For this review, take the finished solid that the model builds, in its own axes (mm). Round coordinates to 2 decimals unless told otherwise and drop trailing zeros. Loops run counter-clockwise (first coordinate to the right, second up) from the corner with the lowest first, then second, coordinate; pieces in that order, holes last. Notation, with made-up numbers: (-22, 18.25) -> (-17, 18.25) arc R33 cw to (-17, 47.25) -> close; hole circle Ø8 at (81, 78). An arc over 180 degrees is marked (long way). Use one line per item in the form item = value. Start each with the question number.
from build123d import *

# Parameters (mm, degrees)
F0_R     = 2.5019
F1_DEPTH = 5.6642


with BuildPart() as f1:
    # F0 (on Front) → F1 (new body)
    with BuildSketch(Plane.XZ):
        with BuildLine():
            Line((62.201412, 5.162847), (-22.03138, 5.162847))
            Line((-22.03138, 5.162847), (-22.38087, 5.162847))
            ThreePointArc((-22.38087, 5.162847), (-27.365937, -0.248725), (-21.883471, -5.155717))
            Line((-21.883471, -5.155717), (62.381241, -5.166))
            ThreePointArc((62.381241, -5.166), (67.547089, 0.089928), (62.201412, 5.162847))
        make_face()
        with Locations((-22.206125, 0)):
            Circle(F0_R, mode=Mode.SUBTRACT)
        with Locations((62.381871, 0)):
            Circle(F0_R, mode=Mode.SUBTRACT)
    extrude(amount=F1_DEPTH)


solid = f1.part
Item 1: Draft analysis for pull direction X (two halves, no side actions). For faces 1 (the cylindrical face through (59.882, -2.792, 0.11)), 2 (the flat face through (19, -5.664, 0)), state which applies: +X half, -X half, draft (parallel to the pull), parting line (faces both ways), or undercut.
Item 2: Take a section at C-C on z = 3.75. Give the boundary of the cut face in (x, y), plus the area to 3 significant figures.
Item 3: Take a section at B-B on y = -3.8. Give the boundary of the cut face in (x, z).
Item 4: For P1, Ø2, axis at y = -4, z = -3.5, coming from the -X side, flat-tipped, find the tip position at first contact; note if it passes through.
Item 5: Wall thickness on line 1 (X direction, y = -4.15, z = 1.5); line 2 (X direction, y = -2.7, z = 0.5); line 3 (Z direction, x = 4, y = -4.3): over which ranges is each line inside the solid? List them lowest first.
Item 6: Take a section at A-A on z = 0. Give the boundary of the cut face in (x, y), plus the area to 3 significant figures.
Results:
q1.face_1 = undercut
q1.face_2 = draft
q2.outline = (-25.76, -5.66) -> (65.94, -5.66) -> (65.94, 0) -> (-25.76, 0) -> close
q2.area = 519 mm2
q3.outline = (-22.38, 5.16) arc R5.17 ccw (long way) to (-21.88, -5.16) -> (62.38, -5.17) arc R5.17 ccw (long way) to (62.2, 5.16) -> close; hole circle Ø5 at (-22.21, 0); hole circle Ø5 at (62.38, 0)
q4.P1 = -26.73
q5.line_1 = -27.15 to -24.21, -20.2 to 60.38, 64.38 to 67.33
q5.line_2 = -27.35 to -24.66, -19.75 to 59.93, 64.83 to 67.52
q5.line_3 = -5.16 to 5.16
q6.outline = (-27.37, -5.66) -> (-24.71, -5.66) -> (-24.71, 0) -> (-27.37, 0) -> close; (-19.7, -5.66) -> (59.88, -5.66) -> (59.88, 0) -> (-19.7, 0) -> close; (64.88, -5.66) -> (67.55, -5.66) -> (67.55, 0) -> (64.88, 0) -> close
q6.area = 481 mm2
